Geometry: final body of the model. Coordinates: model frame, mm. A direction names the side the tool comes from. Coordinates: 2 decimals unless noted, no trailing zeros. Write each loop counter-clockwise with the first axis right and the second up, starting at its lowest first coordinate (ties: lowest second). Pieces come first, ordered by that corner, then holes.
from build123d import *

# Parameters (mm, degrees)
BOSS_EXTRUDE1_DEPTH = 21
CUT_EXTRUDE1_DEPTH  = 22.662179022
BOSS_EXTRUDE2_DEPTH = 49
FILLET1_R           = 0.4
SKETCH4_W           = 7.390362968
SKETCH4_H           = 6.925637862
CUT_EXTRUDE2_DEPTH  = 4.5
CUT_EXTRUDE3_DEPTH  = 66.709283971


with BuildPart() as part:
    # Sketch1 → Boss-Extrude1 (new body)
    with BuildSketch(Plane.XY):
        Polygon((0, 0), (2, 0), (2, 2), (3.5, 2), (3.5, -4), (2, -4), (2, -2), (0, -2), (0, -4), (-1.5, -4), (-1.5, 2), (0, 2), align=None)
    extrude(amount=BOSS_EXTRUDE1_DEPTH)

    # Sketch2 → Cut-Extrude1 (cut, through all)
    with BuildSketch(Plane.XY.offset(21)):
        Polygon((-1.5, 2), (-1.5, 1.9), (-0.1, 1.9), (-0.1, -0.1), (2.1, -0.1), (2.1, 1.9), (3.5, 1.9), (3.5, 2), align=None)
        Polygon((-1.5, -4), (3.5, -4), (3.5, -3.9), (2.1, -3.9), (2.1, -1.9), (-0.1, -1.9), (-0.1, -3.9), (-1.5, -3.9), align=None)
    extrude(amount=-CUT_EXTRUDE1_DEPTH, mode=Mode.SUBTRACT)

    # Sketch3 → Boss-Extrude2 (add)
    with BuildSketch(Plane(origin=(0, 0, 0), x_dir=(-1, 0, 0), z_dir=(0, 0, -1))):
        Polygon((-2.1, -0.1), (-2.1, 1.9), (-3.5, 1.9), (-3.5, -3.9), (-2.1, -3.9), (-2.1, -1.9), (0.1, -1.9), (0.1, -3.9), (1.5, -3.9), (1.5, 1.9), (0.1, 1.9), (0.1, -0.1), align=None)
    extrude(amount=BOSS_EXTRUDE2_DEPTH)

    # Fillet1
    fillet1_edges = [part.edges().sort_by_distance(p)[0] for p in [
        (3.5, 1.9, -14),
        (2.1, 1.9, -14),
        (-0.1, 1.9, -14),
        (-1.5, 1.9, -14),
        (-1.5, -3.9, -14),
        (-0.1, -3.9, -14),
        (2.1, -3.9, -14),
        (3.5, -3.9, -14),
    ]]
    fillet(fillet1_edges, radius=FILLET1_R)

    # Sketch4 → Cut-Extrude2 (cut)
    with BuildSketch(Plane.XY.offset(21)):
        with Locations((1.359853511, -0.992123471)):
            Rectangle(SKETCH4_W, SKETCH4_H)
    extrude(amount=-CUT_EXTRUDE2_DEPTH, mode=Mode.SUBTRACT)

    # Sketch5 → Cut-Extrude3 (cut, through all)
    with BuildSketch(Plane.XY.offset(16.5)):
        Polygon((1, -0.1), (1, -4.471305572), (4.036871247, -4.471305572), (4.036871247, 2.64231625), (1, 2.64231625), align=None)
    extrude(amount=-CUT_EXTRUDE3_DEPTH, mode=Mode.SUBTRACT)


solid = part.part
Item 1: Section C-C, the plane x = 0.4. Output: boundary loops of the cut face in (y, z), plus the area to 3 significant figures.
Derived:
outline: (-1.9, -49) - (-0.1, -49) - (-0.1, 16.5) - (-1.9, 16.5) - close
area: 118 mm2
Item 2: Set-up query: faces 1 (the flat face through (-0.1, 1, -16)), 2 (the flat face through (1, -1, -16)), 3 (the flat face through (0.5, -1.9, -15.8)). Return all of +Z, -Z, +X, -X, +Y, -Y with unobstructed straight access to the full face (end or side cutting, diameter ignored); none if empty.
Derived:
face 1: +Z, -Z, +X, +Y
face 2: +Z, -Z, +X, +Y, -Y
face 3: +Z, -Z, +X, -Y
Item 3: Pin query (flat end, axial travel): pin 1 (1.3 mm diameter, centred on y = 1, z = -17, fed in from +X); pin 2 (0.6 mm diameter, centred on x = 0.5, z = -13, fed in from +Y). Return the tip coordinate at first contact, or that it passes through.
Derived:
pin 1: stops at x = -0.1
pin 2: stops at y = -0.1
Item 4: Material intervals for probe 1 along Y at (x, z) = (-0.4, 12); probe 2 along Y at (x, z) = (0.5, -41); probe 3 along X at (y, z) = (-3.45, -22.5), sorted ascending.
Derived:
probe 1: y = -3.89 to 1.89
probe 2: y = -1.9 to -0.1
probe 3: x = -1.5 to -0.1
Item 5: Section B-B, the plane y = -2.55. Output: boundary loops of the cut face in (x, z), plus the area to 3 significant figures.
Derived:
outline: (-1.5, -49) - (-0.1, -49) - (-0.1, 16.5) - (-1.5, 16.5) - close
area: 91.7 mm2
Item 6: Section A-A, the plane z = -28.5. Output: boundary loops of the cut face in (x, y), plus the area to 3 significant figures.
Derived:
outline: (-1.5, -3.5) arc R0.4 ccw to (-1.1, -3.9) - (-0.5, -3.9) arc R0.4 ccw to (-0.1, -3.5) - (-0.1, -1.9) - (1, -1.9) - (1, -0.1) - (-0.1, -0.1) - (-0.1, 1.5) arc R0.4 ccw to (-0.5, 1.9) - (-1.1, 1.9) arc R0.4 ccw to (-1.5, 1.5) - close
area: 9.96 mm2
